```python
from build123d import *

# Parameters (mm, degrees)
SKETCH_1_R      = 2.25
SKETCH_1_R_2    = 1.75
EXTRUDE_1_DEPTH = 1
SKETCH_3_R      = 1.125
SKETCH_3_R_2    = 0.75
EXTRUDE_2_DEPTH = 8


with BuildPart() as part:
    # 草图1 → 凸台-拉伸1 (new body)
    with BuildSketch(Plane(origin=(0, 0, 0), x_dir=(1, 0, 0), z_dir=(0, 1, 0))):
        Circle(SKETCH_1_R)
        Circle(SKETCH_1_R_2, mode=Mode.SUBTRACT)
    extrude(amount=EXTRUDE_1_DEPTH)

    # 草图2 → 旋转1 (revolve)
    with BuildSketch(Plane(origin=(0, 0, 0), x_dir=(0, 0, -1), z_dir=(1, 0, 0))):
        with BuildLine():
            Line((0, 1), (0, 3.25))
            ThreePointArc((0, 3.25), (-1.590990258, 2.590990258), (-2.25, 1))
            Line((-2.25, 1), (0, 1))
        make_face()
    revolve(axis=Axis((0, 0, 0), (0, 1, 0)))

    # 草图3 → 凸台-拉伸2 (add)
    with BuildSketch(Plane(origin=(0, 0, 0), x_dir=(0, 0, -1), z_dir=(1, 0, 0))):
        with Locations((0, 2.125)):
            Circle(SKETCH_3_R)
        with Locations((0, 2.125)):
            Circle(SKETCH_3_R_2, mode=Mode.SUBTRACT)
    extrude(amount=EXTRUDE_2_DEPTH)


solid = part.part
```
Can you work these out from the model? Positions are in its coordinate system, mm. A direction names the side the tool comes from. Round coordinates to 2 decimals unless told otherwise and drop trailing zeros. Order: outer loops, then holes, each group sorted by start corner. A loop starts at its lowest first (then second) coordinate and runs counter-clockwise, first axis right, second up.
(1) If I drill on L1, parallel to Z at x = 0, y = 0.3; L2, parallel to Y at x = 5, z = 0 (3 decimals), over which ranges is the centre line in solid material (lowest first)?
Results are:
L1: z = -2.25 to -1.75, 1.75 to 2.25
L2: y = 1 to 1.375, 2.875 to 3.25
(2) I'm going to push flat-ended pins straight in: pin 1 (0.9 mm diameter, centred on y = 2.125, z = 0, fed in from +X); pin 2 (2 mm diameter, centred on x = 0, z = 0, fed in from -Y); pin 3 (2 mm diameter, centred on x = 3, z = -0.5, fed in from -Y); pin 4 (1 mm diameter, centred on x = 4.5, y = 1, fed in from +Z). Where does each tip first touch, or does it pass through?
Results are:
pin 1: stops at x = 2.15
pin 2: stops at y = 1
pin 3: stops at y = 0
pin 4: stops at z = 0.94
(3) We'd pull the mould along X, two halves only. Please class faces 1 (the face through (1.617, 0.493, 0.67)), 2 (the face through (4.57, 2.87, 0.1)), 3 (the face through (-0.29, 0.49, -2.23)): +X half, -X half, draft (parallel to the pull), parting line (faces both ways), or undercut.
Results are:
face 1: undercut
face 2: draft
face 3: parting line
(4) If we section it at A-A (x = 2): Please give me the cut outline in (y, z) (3 decimals), plus the area to 3 significant figures.
Results are:
outline: (0, -1.031) - (1, -1.031) arc R1.031 ccw to (1.472, -0.916) arc R1.125 ccw (long way) to (1.472, 0.916) arc R1.031 ccw to (1, 1.031) - (0, 1.031) - close; hole (1.785, -0.668) arc R0.75 ccw (long way) to (1.785, 0.668) arc R1.031 cw to start
area: 5.22 mm2
(5) On a 3-axis mill with a long thin cutter (end or side, diameter ignored), from which of +Z, -Z, +X, -X, +Y, -Y can I reach the whole of each face in a straight line? I mean faces 4 (the face through (4.83, 3.24, 0.15)), 5 (the face through (0, 0, 2)), 6 (the face through (0, 1, 0)). Say none if no direction works.
Results are:
face 4: +X
face 5: +Z, -Z, +X, -X, -Y
face 6: -Y
(6) If we section it at D-D (y = 2.55): Please give me the cut outline in (x, z) (3 decimals), plus the area to 3 significant figures.
Results are:
outline: (1.255, -1.042) - (8, -1.042) - (8, -0.618) - (1.509, -0.618) arc R1.631 ccw to (1.509, 0.618) - (8, 0.618) - (8, 1.042) - (1.255, 1.042) arc R1.631 ccw (long way) to start
area: 14.0 mm2
(7) If we section it at C-C (z = -1.4): Please give me the cut outline in (x, y).
Results are:
outline: (-1.76, 0) - (-1.05, 0) - (-1.05, 1) - (1.05, 1) - (1.05, 0) - (1.76, 0) - (1.76, 1) arc R1.76 ccw to (-1.76, 1) - close
(8) If we section it at B-B (y = 0.3): Please give me the cut outline in (x, z).
Results are:
outline: circle Ø4.5 at (0, 0); hole circle Ø3.5 at (0, 0)
